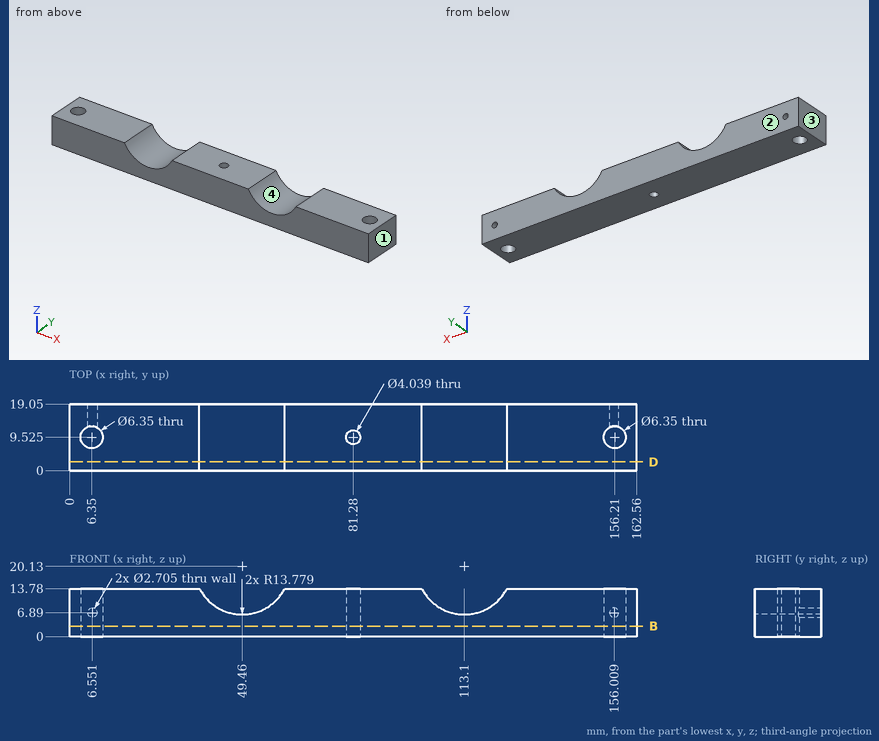
Print and shaded views of the part. All mm, measured from the part's lowest x, y and z. Round coordinates to 2 decimals unless told otherwise and drop trailing zeros. Write each loop counter-clockwise with the first axis right and the second up, starting at its lowest first coordinate (ties: lowest second). Pieces come first, ordered by that corner, then holes.
(1) Probe line 1 along Y through (x, z) = (6.35, 9.75); line 2 along X through (y, z) = (7.75, 11) (1 decimal); line 3 along X through (y, z) = (15.25, 12.75) (1 decimal). List the from-to ranges inside material, lowest first.
(2) Mould opens along X. For the marked faces 1, 2, 3 and 4 say: pulls with the +X half, pulls with the -X half, needs draft (parallel to the pull), parting line crosses it, or undercut.
(3) Drop flat-ended pins along their axis: P1, Ø2.5, axis at x = 81.28, y = 9.525, coming from the +Z side; P2, Ø6, axis at x = 58.5, y = 10.5, coming from the +Z side (1 decimal). Give the stop position or say it passes through.
(4) Slice it at B-B, the plane z = 3. Count the separate pieces of the cut face and the enclosed holes in it, and give its area (3 significant figures).
(5) Slice it at D-D, the plane y = 2.5. Write the cut outline in (x, z).
From the geometry:
1. line 1: y = 0 to 6.35, 12.7 to 19.05
1. line 2: x = 0 to 3.7, 9 to 39.1, 59.8 to 80.3, 82.2 to 102.8, 123.4 to 153.6, 158.8 to 162.6
1. line 3: x = 0 to 37.8, 61.1 to 101.5, 124.7 to 162.6
2. face 1: pulls with the +X half
2. face 2: needs draft
2. face 3: pulls with the -X half
2. face 4: undercut
3. P1: passes through
3. P2: stops at z = 13.4
4. separate pieces: 1
4. enclosed holes: 3
4. area: 3,020 mm2
5. outline: (0, 0) - (162.56, 0) - (162.56, 13.78) - (125.33, 13.78) arc R13.78 cw to (100.87, 13.78) - (61.69, 13.78) arc R13.78 cw to (37.23, 13.78) - (0, 13.78) - close
